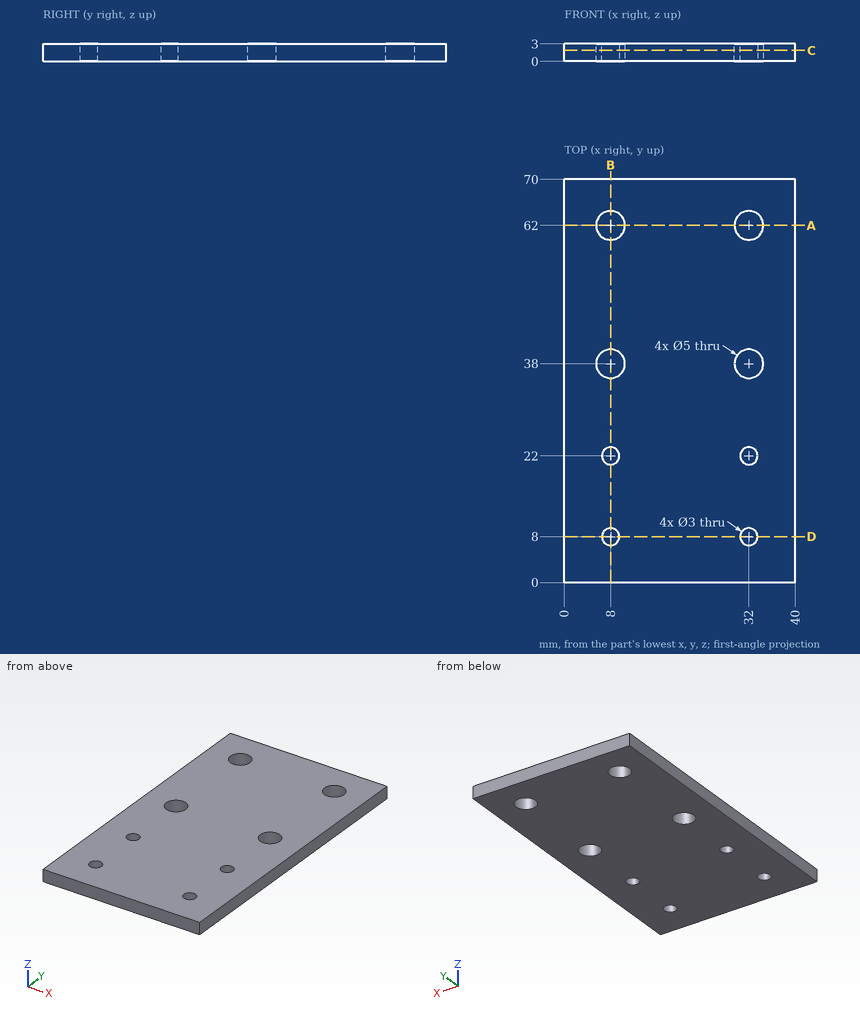
Here's the drawing with two shaded views (mm, measured from the low corner). I have some questions. Give positions to 0.01 mm unless a question says otherwise; leave off trailing zeros. Loops run counter-clockwise (first coordinate to the right, second up) from the corner with the lowest first, then second, coordinate; pieces in that order, holes last. Notation, with made-up numbers: M 52,47.5 L 108,47.5 A28 ccw 108,80.5 Z; hole C 58,44 d6. An arc over 180 degrees is marked long. Answer in a Markdown table with one row per item.
1. Suppose I cut it at D-D on y = 8. Write out the boundary of the cut face in (x, z).
Taken from the geometry:
| item | result |
|---|---|
| outline | M 0,0 L 6.5,0 L 6.5,3 L 0,3 Z; M 9.5,0 L 30.5,0 L 30.5,3 L 9.5,3 Z; M 33.5,0 L 40,0 L 40,3 L 33.5,3 Z |
2. If I drill on line 1 along Y through (x, z) = (32, 0.65); line 2 along X through (y, z) = (60, 0.45); line 3 along X through (y, z) = (8.5, 1.2), over which ranges is the centre line in solid material (lowest first)?
Taken from the geometry:
| item | result |
|---|---|
| line 1 | y = 0 to 6.5, 9.5 to 20.5, 23.5 to 35.5, 40.5 to 59.5, 64.5 to 70 |
| line 2 | x = 0 to 6.5, 9.5 to 30.5, 33.5 to 40 |
| line 3 | x = 0 to 6.59, 9.41 to 30.59, 33.41 to 40 |
3. For pin 1 Ø4 at (x, y) = (32, 8) entering from -Z, with a flat end and sliding along its axis, tell me the tip position at first contact or that it passes through.
Taken from the geometry:
| item | result |
|---|---|
| pin 1 | stops at z = 0 |
4. Suppose I cut it at B-B on x = 8. Write out the boundary of the cut face in (y, z), plus the area to 3 significant figures.
Taken from the geometry:
| item | result |
|---|---|
| outline | M 0,0 L 6.5,0 L 6.5,3 L 0,3 Z; M 9.5,0 L 20.5,0 L 20.5,3 L 9.5,3 Z; M 23.5,0 L 35.5,0 L 35.5,3 L 23.5,3 Z; M 40.5,0 L 59.5,0 L 59.5,3 L 40.5,3 Z; M 64.5,0 L 70,0 L 70,3 L 64.5,3 Z |
| area | 162 mm² |
5. Suppose I cut it at C-C on z = 1.9. Count the separate pieces of the cut face and the enclosed holes in it, plus the area to 3 significant figures.
Taken from the geometry:
| item | result |
|---|---|
| separate pieces | 1 |
| enclosed holes | 8 |
| area | 2,690 mm² |
6. Suppose I cut it at A-A on y = 62. Write out the boundary of the cut face in (x, z), plus the area to 3 significant figures.
Taken from the geometry:
| item | result |
|---|---|
| outline | M 0,0 L 5.5,0 L 5.5,3 L 0,3 Z; M 10.5,0 L 29.5,0 L 29.5,3 L 10.5,3 Z; M 34.5,0 L 40,0 L 40,3 L 34.5,3 Z |
| area | 90.0 mm² |
